Geometry check sheet. Reference: the model listing, model coordinates, mm. Face numbers are marked on the shaded views. A direction names the side the tool comes from. Give positions to 0.01 mm unless a question says otherwise; leave off trailing zeros. Write each loop counter-clockwise with the first axis right and the second up, starting at its lowest first coordinate (ties: lowest second). Pieces come first, ordered by that corner, then holes. Notation, with made-up numbers: (38.5, 80) -> (70.5, 80) arc R21 ccw to (70.5, 88) -> close; hole circle Ø4 at (-6, 18.25). An arc over 180 degrees is marked (long way). Write item = value, one per line. Start each with the question number.
1. Cross-section at A-A, the plane x = 0. Record the cut outline in (y, z).
2. Depth check by flat-ended pin: P1, Ø8, axis at x = 7.5, z = 7.5, coming from the -Y side; P2, Ø1, axis at y = 2.5, z = 2.5, coming from the -X side; P3, Ø5, axis at x = 9.5, y = 1, coming from the -Z side. Enter the tip coordinate at first touch or a pass-through.
3. Set-up check for the marked faces 1 and 2: record each of +Z, -Z, +X, -X, +Y, -Y from which the full face is reachable in a straight line by a thin tool's end or side.
4. Cross-section at D-D, the plane x = 4.5. Record the cut outline in (y, z).
5. Thickness scan on line 1 along Y through (x, z) = (10, 1.6); line 2 along Z through (x, y) = (11.5, -3.25); line 3 along X through (y, z) = (-2, 10.25). Record the ranges inside material, lowest first.
6. Cross-section at B-B, the plane z = 6. Record the cut outline in (x, y), plus the area to 3 significant figures.
7. Cross-section at C-C, the plane y = 3.5. Record the cut outline in (x, z).
```python
from build123d import *

# Parameters (mm, degrees)
F1_DEPTH       = 3
F2_D           = 0.34
F2_DEPTH       = 2
F2_CSINK_D     = 0.63
F2_CSINK_ANGLE = 90
F2_TIP         = 0.1021463052
F5_R           = 2.5
F6_DEPTH       = 14


# Not quite as in the source:
# - the program builds the solid bodies; features that only make, move or delete a surface that nothing else refers to are left out


with BuildPart() as f1:
    # F0 (on Top) → F1 (new body)
    with BuildSketch(Plane.XY):
        with BuildLine():
            Line((13.2871780876, 4.4103172753), (-13.2871780876, 4.4103172753))
            ThreePointArc((-13.2871780876, 4.4103172753), (-14, 0), (-13.2871780876, -4.4103172753))
            Line((-13.2871780876, -4.4103172753), (13.2871780876, -4.4103172753))
            ThreePointArc((13.2871780876, -4.4103172753), (14, 0), (13.2871780876, 4.4103172753))
        make_face()
    extrude(amount=F1_DEPTH)

    # F2
    with Locations(Plane(origin=(0, 0, 0), x_dir=(1, 0, 0), z_dir=(0, 0, -1))):
        with Locations((-10, 0), (10, 0)):
            CounterSinkHole(F2_D / 2, F2_CSINK_D / 2, depth=F2_DEPTH, counter_sink_angle=F2_CSINK_ANGLE)
            with Locations((0, 0, -(F2_DEPTH + F2_TIP / 2))):  # 118° drill point
                Cone(0, F2_D / 2, F2_TIP, mode=Mode.SUBTRACT)

    # F5 (on Top) → F6 (join)
    with BuildSketch(Plane.XY):
        Circle(F5_R)
    extrude(amount=F6_DEPTH)


solid = f1.part
```
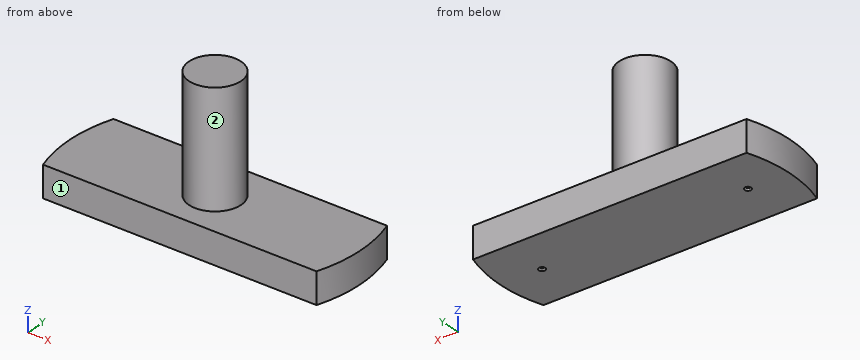
Answers:
q1.outline = (-4.41, 0) -> (4.41, 0) -> (4.41, 3) -> (2.5, 3) -> (2.5, 14) -> (-2.5, 14) -> (-2.5, 3) -> (-4.41, 3) -> close
q2.P1 = through
q2.P2 = -13.86
q2.P3 = 0
q3.face_1 = +Z, -Z, +X, -X, -Y
q3.face_2 = +Z
q4.outline = (-4.41, 0) -> (4.41, 0) -> (4.41, 3) -> (-4.41, 3) -> close
q5.line_1 = -4.41 to -0.17, 0.17 to 4.41
q5.line_2 = 0 to 3
q5.line_3 = -1.5 to 1.5
q6.outline = circle Ø5 at (0, 0)
q6.area = 19.6 mm^2
q7.outline = (-13.56, 0) -> (13.56, 0) -> (13.56, 3) -> (-13.56, 3) -> close
